from build123d import *

# Parameters (mm, degrees)
ESQUISSE1_W             = 16
ESQUISSE1_H             = 28.5
BOSS_EXTRU_1_DEPTH      = 8
ENL_V_MAT_EXTRU_1_DEPTH = 5.5
ESQUISSE3_R             = 2.5
ENL_V_MAT_EXTRU_2_DEPTH = 3.5
ESQUISSE4_W             = 7.5
ESQUISSE4_H             = 8
BOSS_EXTRU_2_DEPTH      = 10
CHANFREIN2_SIZE         = 3
ESQUISSE5_R             = 2.5
ENL_V_MAT_EXTRU_3_DEPTH = 9
CONG_1_R                = 3


with BuildPart() as part:
    # Esquisse1 → Boss.-Extru.1 (new body)
    with BuildSketch(Plane(origin=(0, 0, 0), x_dir=(0, 0, -1), z_dir=(1, 0, 0))):
        Rectangle(ESQUISSE1_W, ESQUISSE1_H)
    extrude(amount=BOSS_EXTRU_1_DEPTH)

    # Esquisse2 → Enlèv. mat.-Extru.1 (cut)
    with BuildSketch(Plane(origin=(8, 0, 0), x_dir=(0, 0, -1), z_dir=(1, 0, 0))):
        Polygon((4.041451884, 8.25), (2.020725942, 11.75), (-2.020725942, 11.75), (-4.041451884, 8.25), (-2.020725942, 4.75), (2.020725942, 4.75), align=None)
    extrude(amount=-ENL_V_MAT_EXTRU_1_DEPTH, mode=Mode.SUBTRACT)

    # Esquisse3 → Enlèv. mat.-Extru.2 (cut, through all)
    with BuildSketch(Plane(origin=(2.5, 0, 0), x_dir=(0, 0, -1), z_dir=(1, 0, 0))):
        with Locations((0, 8.25)):
            Circle(ESQUISSE3_R)
    extrude(amount=-ENL_V_MAT_EXTRU_2_DEPTH, mode=Mode.SUBTRACT)

    # Esquisse4 → Boss.-Extru.2 (add)
    with BuildSketch(Plane(origin=(8, 0, 0), x_dir=(0, 0, -1), z_dir=(1, 0, 0))):
        with Locations((0, -2.75)):
            Rectangle(ESQUISSE4_W, ESQUISSE4_H)
    extrude(amount=BOSS_EXTRU_2_DEPTH)

    # Chanfrein2
    chanfrein2_edges = [part.edges().sort_by_distance(p)[0] for p in [
        (13, 1.25, -3.75),
        (13, 1.25, 3.75),
    ]]
    chamfer(chanfrein2_edges, length=CHANFREIN2_SIZE)

    # Symétrie1: part across plane


with BuildPart() as part_1:
    add(part.part)
    add(part.part.mirror(Plane(origin=(8, -14.25, 8), x_dir=(0, 0, 1), z_dir=(0, 1, 0))))

    # Esquisse5 → Enlèv. mat.-Extru.3 (cut, through all)
    with BuildSketch(Plane(origin=(8, 0, 0), x_dir=(0, 0, -1), z_dir=(1, 0, 0))):
        with Locations((0, -14.25)):
            Circle(ESQUISSE5_R)
    extrude(amount=-ENL_V_MAT_EXTRU_3_DEPTH, mode=Mode.SUBTRACT)

    # Congé1
    cong_1_edges = [part_1.edges().sort_by_distance(p)[0] for p in [
        (4, 14.25, 8),
        (4, 14.25, -8),
    ]]
    fillet(cong_1_edges, radius=CONG_1_R)


solid = part_1.part
Input: part model. Units: mm. Frame: model coordinates. A direction names the side the tool comes from. Coordinates: 2 decimals unless noted, no trailing zeros. Loops run counter-clockwise (first coordinate to the right, second up) from the corner with the lowest first, then second, coordinate; pieces in that order, holes last.
Q1. Set-up query: faces 1 (the face through (13, 0, -2)), 2 (the face through (5.288, 9.976, -3.045)), 3 (the face through (13, 0, 2)), 4 (the face through (13, -29.75, 0)). Return all of +Z, -Z, +X, -X, +Y, -Y with unobstructed straight access to the full face (end or side cutting, diameter ignored); none if empty.
Q2. Contact query for flat-ended pins moving along their axis: pin 1 (2.5 mm diameter, centred on x = 15.5, y = -4.5, fed in from -Z); pin 2 (3 mm diameter, centred on x = 8.5, z = -3.5, fed in from -Y); pin 3 (1.2 mm diameter, centred on x = 15.5, z = 0, fed in from +Y); pin 4 (2 mm diameter, centred on x = 10, z = -1.5, fed in from -Y). Output: stop coordinate, or through.
Q3. Cut plane A-A (x = 9.5). Output: boundary loops of the cut face in (y, z), then the cut area to 3 significant figures.
Q4. Cut plane C-C (z = 0). Give the number of separate pieces and of enclosed holes in the cut face, then the cut area to 3 significant figures.
Q5. Material intervals for line 1 (Y direction, x = 0.55, z = 0); line 2 (Y direction, x = 3, z = 0); line 3 (Z direction, x = 1, y = -36.75), sorted ascending.
Q6. Cut plane D-D (x = 1.5). Output: boundary loops of the cut face in (y, z), then the cut area to 3 significant figures.
Q7. Draft query along Z for faces 5 (the face through (12.9, -28.2, 2.3)), 6 (the face through (4.1, -16.7, 0.5)), 7 (the face through (4, -15, -8)), 8 (the face through (13, 1.25, 0)). Return one class per face: +Z half, -Z half, draft (parallel to the pull), parting line (faces both ways), or undercut.
Q8. Cut plane B-B (y = -14.25). Output: boundary loops of the cut face in (x, z).
Working result:
1. face 1: -Z, +X, +Y
1. face 2: +X
1. face 3: +Z, +X, +Y
1. face 4: +Z, -Z, +X, -Y
2. pin 1: stops at z = -3.75
2. pin 2: stops at y = -42.75
2. pin 3: stops at y = 1.25
2. pin 4: stops at y = -29.75
3. outline: (-29.75, -0.75) - (-26.75, -3.75) - (-21.75, -3.75) - (-21.75, 3.75) - (-26.75, 3.75) - (-29.75, 0.75) - close; (-6.75, -3.75) - (-1.75, -3.75) - (1.25, -0.75) - (1.25, 0.75) - (-1.75, 3.75) - (-6.75, 3.75) - close
3. area: 102 mm2
4. separate pieces: 4
4. enclosed holes: 0
4. area: 474 mm2
5. line 1: y = -42.75 to -39.25, -34.25 to -16.75, -11.75 to 5.75, 10.75 to 14.25
5. line 2: y = -42.75 to -40.25, -33.25 to -16.75, -11.75 to 4.75, 11.75 to 14.25
5. line 3: z = -8 to -2.5, 2.5 to 8
6. outline: (-42.75, -8) - (11.25, -8) arc R3 ccw to (14.25, -5) - (14.25, 5) arc R3 ccw to (11.25, 8) - (-42.75, 8) - close; hole circle Ø5 at (-36.75, 0); hole circle Ø5 at (-14.25, 0); hole circle Ø5 at (8.25, 0)
6. area: 849 mm2
7. face 5: +Z half
7. face 6: undercut
7. face 7: -Z half
7. face 8: draft
8. outline: (0, -8) - (8, -8) - (8, -2.5) - (0, -2.5) - close; (0, 2.5) - (8, 2.5) - (8, 8) - (0, 8) - close
